Source: CAD feature listing. Evaluate the final solid. Frame: model axes, mm. A direction names the side the tool comes from. Give positions to 0.01 mm unless a question says otherwise; leave off trailing zeros. Write each loop counter-clockwise with the first axis right and the second up, starting at its lowest first coordinate (ties: lowest second). Pieces come first, ordered by that corner, then holes.
```python
from build123d import *

# Parameters (mm, degrees)
SKETCH1_W           = 41.656
SKETCH1_H           = 60.855895471
BOSS_EXTRUDE1_DEPTH = 10.905899582
CUT_EXTRUDE1_DEPTH  = 59.321153171
SKETCH5_W           = 2.0193
SKETCH5_H           = 60.855895471
SKETCH6_W           = 2.0193
SKETCH6_H           = 12.7
SKETCH7_W           = 2.0193
SKETCH7_H           = 12.7
SKETCH8_W           = 10.905899582
SKETCH8_H           = 60.855895471
SKETCH8_R           = 2.0193
BOSS_EXTRUDE2_DEPTH = 15.24
SKETCH9_R           = 2.0193
CUT_EXTRUDE2_DEPTH  = 68.202629317


with BuildPart() as part:
    # Sketch1 → Boss-Extrude1 (new body)
    with BuildSketch(Plane(origin=(27.95338, 0, 0), x_dir=(0, 0, -1), z_dir=(1, 0, 0))):
        with Locations((-8.128, -19.008560287)):
            Rectangle(SKETCH1_W, SKETCH1_H)
    extrude(amount=-BOSS_EXTRUDE1_DEPTH)

    # Sketch2 → Cut-Extrude1 (cut, through all)
    with BuildSketch(Plane.ZY.offset(-17.047480418)):
        with BuildLine():
            Line((-12.7, 6.54304), (-12.7, -44.64304))
            Line((-12.7, -44.64304), (0, -44.64304))
            Line((0, -44.64304), (0, -44.560160575))
            ThreePointArc((0, -44.560160575), (5.172627526, -42.4175881), (7.3152, -37.244960575))
            Line((7.3152, -37.244960575), (7.3152, -0.77216))
            ThreePointArc((7.3152, -0.77216), (5.172627526, 4.400467526), (0, 6.54304))
            Line((0, 6.54304), (-12.7, 6.54304))
        make_face()
    extrude(amount=-CUT_EXTRUDE1_DEPTH, mode=Mode.SUBTRACT)

    # Sketch5 → Cut-Revolve3 (revolve, cut)
    with BuildSketch(Plane(origin=(0, 0, -6.35), x_dir=(-1, 0, 0), z_dir=(0, 0, -1)), mode=Mode.PRIVATE) as cut_revolve3_sk:
        with Locations((-23.510080209, -19.008560287)):
            Rectangle(SKETCH5_W, SKETCH5_H)
    revolve(cut_revolve3_sk.sketch.rotate(Axis((22.500430209, -49.436508023, -6.35), (0, 1, 0)), 270), axis=Axis((22.500430209, -49.436508023, -6.35), (0, 1, 0)), mode=Mode.SUBTRACT)

    # Sketch6 → Cut-Revolve4 (revolve, cut)
    with BuildSketch(Plane(origin=(0, -22.756653096, 0), x_dir=(1, 0, 0), z_dir=(0, 1, 0))):
        with Locations((23.510080209, -22.606)):
            Rectangle(SKETCH6_W, SKETCH6_H)
    revolve(axis=Axis((22.500430209, -22.756653096, 16.256), (0, 0, 1)), mode=Mode.SUBTRACT)

    # Sketch7 → Cut-Revolve5 (revolve, cut)
    with BuildSketch(Plane(origin=(0, -15.260467479, 0), x_dir=(1, 0, 0), z_dir=(0, 1, 0))):
        with Locations((23.510080209, -22.606)):
            Rectangle(SKETCH7_W, SKETCH7_H)
    revolve(axis=Axis((22.500430209, -15.260467479, 16.256), (0, 0, 1)), mode=Mode.SUBTRACT)

    # Sketch8 → Boss-Extrude2 (add)
    with BuildSketch(Plane.XY.offset(28.956)):
        with Locations((22.500430209, -19.008560287)):
            Rectangle(SKETCH8_W, SKETCH8_H)
        with Locations((22.500430209, -22.756653096)):
            Circle(SKETCH8_R, mode=Mode.SUBTRACT)
        with Locations((22.500430209, -15.260467479)):
            Circle(SKETCH8_R, mode=Mode.SUBTRACT)
    extrude(amount=BOSS_EXTRUDE2_DEPTH)

    # Sketch9 → Cut-Extrude2 (cut, through all)
    with BuildSketch(Plane(origin=(27.95338, 0, 0), x_dir=(0, 0, -1), z_dir=(1, 0, 0))):
        with Locations((-33.9852, -4.465939121)):
            Circle(SKETCH9_R)
        with Locations((-16.2052, -4.465939121)):
            Circle(SKETCH9_R)
    extrude(amount=-CUT_EXTRUDE2_DEPTH, mode=Mode.SUBTRACT)


solid = part.part
```
1. Mould query, pull axis X, two halves, no side actions, for faces 4 (the flat face through (27.953, -19, 22)), 5 (the flat face through (23, -23, 16.256)), 6 (the flat face through (25, -44.643, -6)). Classes: +X half, -X half, draft (parallel to the pull), parting line (faces both ways), or undercut.
2. Access query for faces 1 (the flat face through (22, -19, 44.196)), 2 (the flat face through (22, -19, 7.315)), 3 (the cylindrical face through (20.483, -15.172, 30.03)). Directions: +Z, -Z, +X, -X, +Y, -Y. A direction counts if a zero-diameter tool reaches every point of the face in a straight line with its end or side. Return the directions, or none.
3. Contact query for flat-ended pins moving along their axis: P1, Ø3, axis at y = -4.47, z = 33.99, coming from the +X side; P2, Ø3.5, axis at x = 20.5, y = -24.5, coming from the -Z side. Output: stop coordinate, or through.
4. Cut plane D-D, the plane y = -27. Return the cut outline in (x, z).
5. Cut plane B-B, the plane z = 35. Return the cut outline in (x, y).
6. Cut plane C-C, the plane x = 18.5. Return the cut outline in (y, z).
7. Cut plane A-A, the plane z = -6.35. Return the cut outline in (x, y), then the cut area to 3 significant figures.
8. Line query: L1, parallel to Y at x = 22.25, z = 19.5; L2, parallel to Y at x = 21.5, z = 30.5; L3, parallel to Y at x = 19.5, z = -7. Output: solid intervals per line, ascending.
Response values:
1. face 4: +X half
1. face 5: undercut
1. face 6: draft
2. face 1: +Z, +X, -X, +Y, -Y
2. face 2: -Z, +X, -X
2. face 3: +Z
3. P1: passes through
3. P2: stops at z = 7.32
4. outline: (17.05, 7.32) - (27.95, 7.32) - (27.95, 44.2) - (17.05, 44.2) - close
5. outline: (17.05, -49.44) - (27.95, -49.44) - (27.95, -6.21) - (17.05, -6.21) - close; (17.05, -2.72) - (27.95, -2.72) - (27.95, 11.42) - (17.05, 11.42) - close; hole circle Ø4.04 at (22.5, -22.76); hole circle Ø4.04 at (22.5, -15.26)
6. outline: (-49.44, -12.7) - (-44.64, -12.7) - (-44.64, 0) - (-44.56, 0) arc R7.32 cw to (-37.24, 7.32) - (-0.77, 7.32) arc R7.32 cw to (6.54, 0) - (6.54, -12.7) - (11.42, -12.7) - (11.42, 44.2) - (-49.44, 44.2) - close; hole circle Ø4.04 at (-4.47, 16.21); hole circle Ø4.04 at (-4.47, 33.99)
7. outline: (17.05, -49.44) - (20.48, -49.44) - (20.48, -44.64) - (17.05, -44.64) - close; (17.05, 6.54) - (20.48, 6.54) - (20.48, 11.42) - (17.05, 11.42) - close; (24.52, -49.44) - (27.95, -49.44) - (27.95, -44.64) - (24.52, -44.64) - close; (24.52, 6.54) - (27.95, 6.54) - (27.95, 11.42) - (24.52, 11.42) - close
7. area: 66.4 mm2
8. L1: y = -49.44 to -24.76, -20.75 to -17.26, -13.26 to 11.42
8. L2: y = -49.44 to -24.51, -21 to -17.01, -13.51 to 11.42
8. L3: y = -49.44 to -44.64, 6.54 to 11.42
